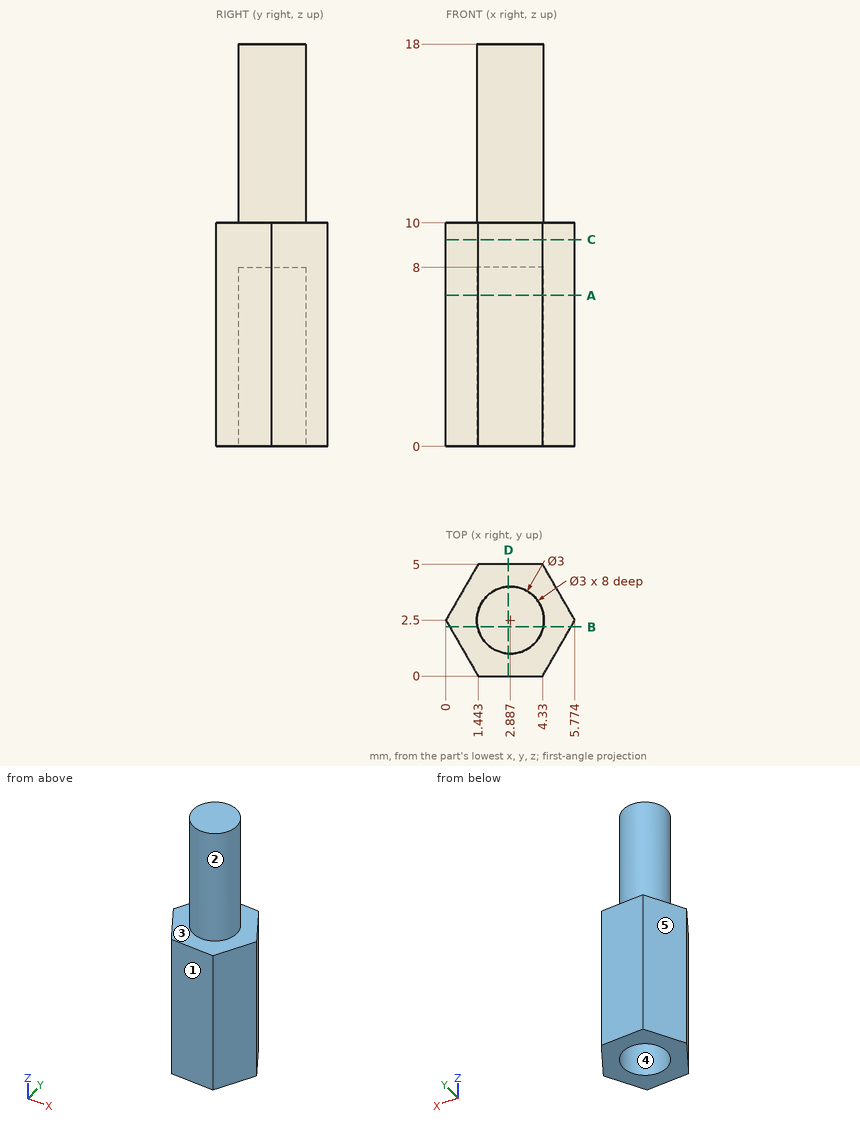
Job drawing, mm, ordinate dimensions from the low corner. One solid piece. A direction names the side the tool comes from. Give positions to 0.01 mm unless a question says otherwise; leave off trailing zeros. Write each loop counter-clockwise with the first axis right and the second up, starting at its lowest first coordinate (ties: lowest second). Pieces come first, ordered by that corner, then holes. Notation, with made-up numbers: (58.5, 89) -> (89.5, 89) arc R13 cw to (89.5, 93) -> close; hole circle Ø5 at (2, -37). An arc over 180 degrees is marked (long way). Return JSON: item names as keys, results as strings.
Item 1: Drop flat-ended pins along their axis: pin 1 (1 mm diameter, centred on y = 3.5, z = 2, fed in from -X); pin 2 (3 mm diameter, centred on x = 3.5, z = 14, fed in from +Y); pin 3 (1 mm diameter, centred on x = 4.5, z = 11.5, fed in from +Y) (1 decimal). Give the stop position or say it passes through.
Answer below:
{"pin 1": "stops at x = 0.29", "pin 2": "stops at y = 4", "pin 3": "stops at y = 3.5"}
Item 2: Drill centre lines: probe 1 along Z at (x, y) = (4.5, 0.6); probe 2 along Z at (x, y) = (4, 2.1); probe 3 along Y at (x, z) = (3, 11.5) (1 decimal). Where is each one in solid material? Low to high.
Answer below:
{"probe 1": "z = 0 to 10", "probe 2": "z = 8 to 18", "probe 3": "y = 1 to 4"}
Item 3: Band-saw the part on C-C (z = 9.25). List the corners of the cut face in (x, y).
Answer below:
{"outline": "(0, 2.5) -> (1.44, 0) -> (4.33, 0) -> (5.77, 2.5) -> (4.33, 5) -> (1.44, 5) -> close"}
Item 4: Band-saw the part on A-A (z = 6.75). List the corners of the cut face in (x, y).
Answer below:
{"outline": "(0, 2.5) -> (1.44, 0) -> (4.33, 0) -> (5.77, 2.5) -> (4.33, 5) -> (1.44, 5) -> close; hole circle Ø3 at (2.89, 2.5)"}
Item 5: Band-saw the part on D-D (x = 2.8). List the corners of the cut face in (y, z).
Answer below:
{"outline": "(0, 0) -> (1, 0) -> (1, 8) -> (4, 8) -> (4, 0) -> (5, 0) -> (5, 10) -> (4, 10) -> (4, 18) -> (1, 18) -> (1, 10) -> (0, 10) -> close"}
Item 6: Two-plate mould, pull along X, no slides. Class the marked faces 3, 4 and 5: +X half, -X half, draft (parallel to the pull), parting line (faces both ways), or undercut.
Answer below:
{"face 3": "draft", "face 4": "undercut", "face 5": "-X half"}
Item 7: Tool access for the marked faces 1 and 2: list every direction of +Z, -Z, +X, -X, +Y, -Y with a clear straight run to the whole face (end or side of a thin tool).
Answer below:
{"face 1": "+Z, -Z, +X, -X, -Y", "face 2": "+Z"}
Item 8: Band-saw the part on B-B (y = 2.2). List the corners of the cut face in (x, z).
Answer below:
{"outline": "(0.17, 0) -> (1.42, 0) -> (1.42, 8) -> (4.36, 8) -> (4.36, 0) -> (5.6, 0) -> (5.6, 10) -> (4.36, 10) -> (4.36, 18) -> (1.42, 18) -> (1.42, 10) -> (0.17, 10) -> close"}
